Here's the drawing with two shaded views (mm, measured from the low corner). I have some questions. Coordinates: 2 decimals unless noted, no trailing zeros. Loops run counter-clockwise (first coordinate to the right, second up) from the corner with the lowest first, then second, coordinate; pieces in that order, holes last. Notation, with made-up numbers: (78.25, 5.25) -> (119.25, 5.25) arc R27 ccw to (119.25, 44.25) -> close; hole circle Ø10 at (69.5, 35). An arc over 180 degrees is marked (long way). Answer as a JSON object with one key per item and string values. Group by question number.
Q1. I want a section at A-A on z = 34.5. Write out the boundary of the cut face in (x, y).
Q2. I want a section at B-B on x = 10. Write out the boundary of the cut face in (y, z).
Q3. I'm going to push flat-ended pins straight in: pin 1 (0.8 mm diameter, centred on y = 0.5, z = 5.5, fed in from +X); pin 2 (0.5 mm diameter, centred on y = 0.5, z = 30.5, fed in from -X). Where does each tip first touch, or does it pass through?
Q4. I want a section at D-D on x = 3. Write out the boundary of the cut face in (y, z), then the cut area to 3 significant figures.
Q5. I need wall thicknesses on line 1 (X direction, y = 0.9, z = 48.5); line 2 (X direction, y = 0.85, z = 5.5) (3 decimals); line 3 (Z direction, x = 24, y = 0.25). Which ranges of each line are inside material? Lowest first, please.
Q6. I want a section at C-C on z = 43. Write out the boundary of the cut face in (x, y).
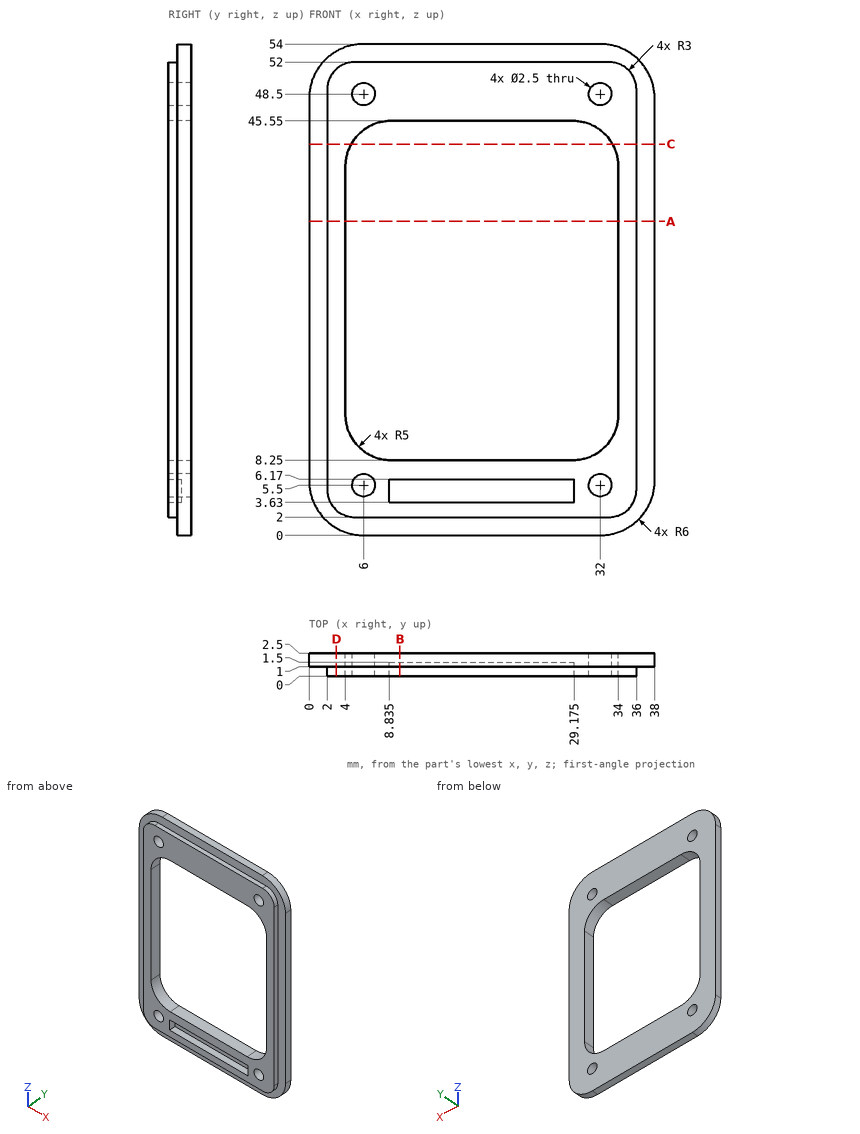
Result set:
{
 "1": {"outline": "(0, 1) -> (2, 1) -> (2, 0) -> (4, 0) -> (4, 2.5) -> (0, 2.5) -> close; (34, 0) -> (36, 0) -> (36, 1) -> (38, 1) -> (38, 2.5) -> (34, 2.5) -> close"},
 "2": {"outline": "(0, 2) -> (1, 2) -> (1, 0) -> (2.5, 0) -> (2.5, 8.25) -> (0, 8.25) -> (0, 6.17) -> (1.5, 6.17) -> (1.5, 3.63) -> (0, 3.63) -> close; (0, 45.55) -> (2.5, 45.55) -> (2.5, 54) -> (1, 54) -> (1, 52) -> (0, 52) -> close"},
 "3": {"pin 1": "stops at x = 36", "pin 2": "stops at x = 2"},
 "4": {"outline": "(0, 2.76) -> (1, 2.76) -> (1, 0.8) -> (2.5, 0.8) -> (2.5, 53.2) -> (1, 53.2) -> (1, 51.24) -> (0, 51.24) -> close", "area": "127 mm²"},
 "5": {"line 1": "x = 2 to 4.75, 7.25 to 30.75, 33.25 to 36", "line 2": "x = 2 to 4.75, 7.25 to 8.835, 29.175 to 30.75, 33.25 to 36", "line 3": "z = 2 to 3.63, 6.17 to 8.25, 45.55 to 52"},
 "6": {"outline": "(0, 1) -> (2, 1) -> (2, 0) -> (4.64, 0) -> (4.64, 2.5) -> (0, 2.5) -> close; (33.36, 0) -> (36, 0) -> (36, 1) -> (38, 1) -> (38, 2.5) -> (33.36, 2.5) -> close"}
}
